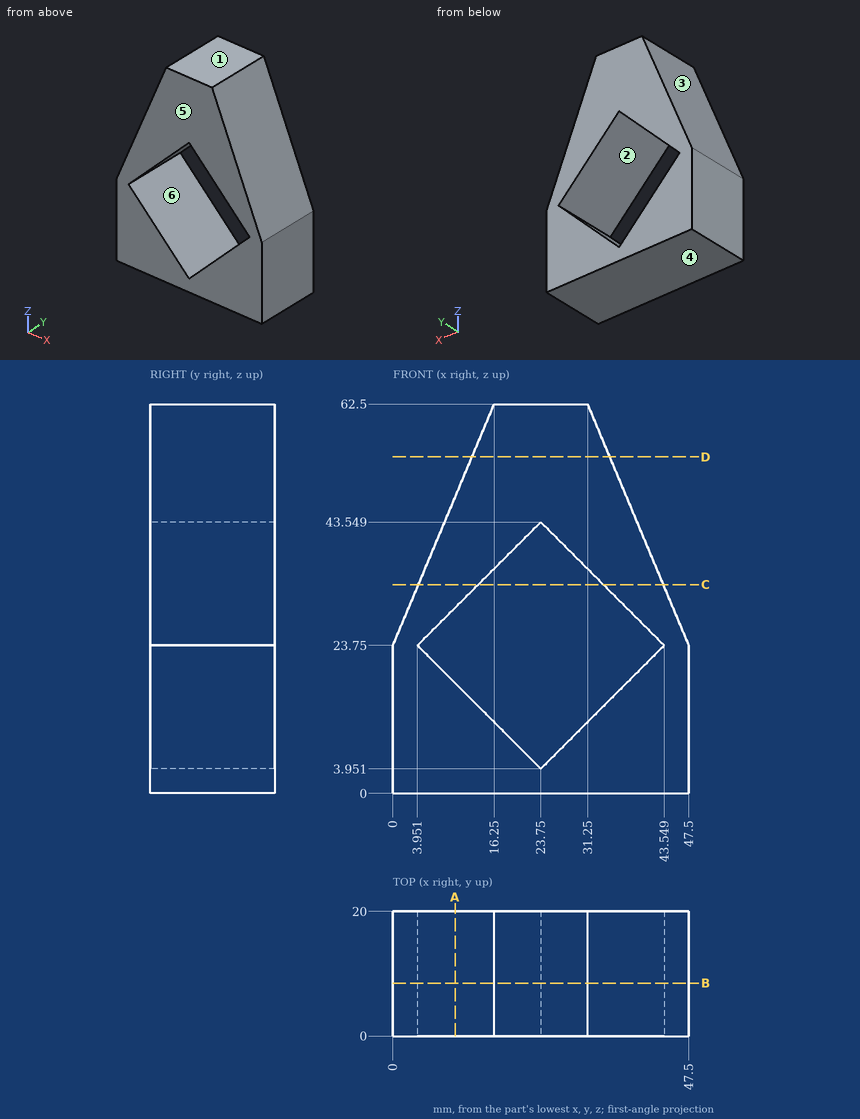
The drawing under review shows one solid part. Ordinate dimensions are in mm from its lowest x, y, z. A direction names the side the tool comes from. Round coordinates to 2 decimals unless told otherwise and drop trailing zeros. Write each loop counter-clockwise with the first axis right and the second up, starting at its lowest first coordinate (ties: lowest second). Pieces come first, ordered by that corner, then holes.
(1) Mouldability with a two-part tool opening along Z and no side actions: class the marked faces 3, 4, 5 and 6 as +Z half, -Z half, draft (parallel to the pull), parting line (faces both ways), or undercut.
(2) Wall thickness on L1, parallel to Z at x = 7, y = 18.75; L2, parallel to Z at x = 6.5, y = 8.25; L3, parallel to X at y = 10.5, z = 6.5: over which ranges is each line inside the solid? List them lowest first.
(3) We need section A-A on x = 10. Give the boundary of the cut face in (y, z), and give its area (3 significant figures).
(4) Machinability: for the marked faces 1 and 2, which of the approach directions +Z, -Z, +X, -X, +Y, -Y give a long, thin tool a straight path to every point of the face, cutting with its end or side? Answer none if there is none.
(5) We need section C-C on z = 33.5. Give the boundary of the cut face in (x, y), and give its area (3 significant figures).
(6) We need section D-D on z = 54. Give the boundary of the cut face in (x, y).
(7) We need section B-B on y = 8.5. Give the boundary of the cut face in (x, z).
(8) Insertion check: pin 1 (1.5 mm diameter, centred on y = 17, z = 31.5, fed in from +X). The pin has a flat end and moves straight along its axis. Give the tip position at first contact, or say it passes through.
Findings below:
1. face 3: +Z half
1. face 4: -Z half
1. face 5: draft
1. face 6: undercut
2. L1: z = 0 to 20.7, 26.8 to 40.44
2. L2: z = 0 to 21.2, 26.3 to 39.25
2. L3: x = 0 to 21.2, 26.3 to 47.5
3. outline: (0, 0) - (20, 0) - (20, 17.7) - (0, 17.7) - close; (0, 29.8) - (20, 29.8) - (20, 47.6) - (0, 47.6) - close
3. area: 710 mm2
4. face 1: +Z, +X, -X, +Y, -Y
4. face 2: +Y, -Y
5. outline: (4.09, 0) - (13.7, 0) - (13.7, 20) - (4.09, 20) - close; (33.8, 0) - (43.41, 0) - (43.41, 20) - (33.8, 20) - close
5. area: 384 mm2
6. outline: (12.69, 0) - (34.81, 0) - (34.81, 20) - (12.69, 20) - close
7. outline: (0, 0) - (47.5, 0) - (47.5, 23.75) - (31.25, 62.5) - (16.25, 62.5) - (0, 23.75) - close; hole (3.95, 23.75) - (23.75, 3.95) - (43.55, 23.75) - (23.75, 43.55) - close
8. pin 1: stops at x = 44.56
